Check sheet for the drawn part. Datum: minimum x, y, z corner. Units: mm. Coordinates: 2 decimals unless noted, no trailing zeros. Order: outer loops, then holes, each group sorted by start corner. A loop starts at its lowest first (then second) coordinate and runs counter-clockwise, first axis right, second up. Notation, with made-up numbers: (16.5, 11) - (69.5, 11) arc R30 ccw to (69.5, 36) - close; hole circle Ø2 at (82.25, -23). An arc over 180 degrees is marked (long way). Put each result on its own line as item: value.
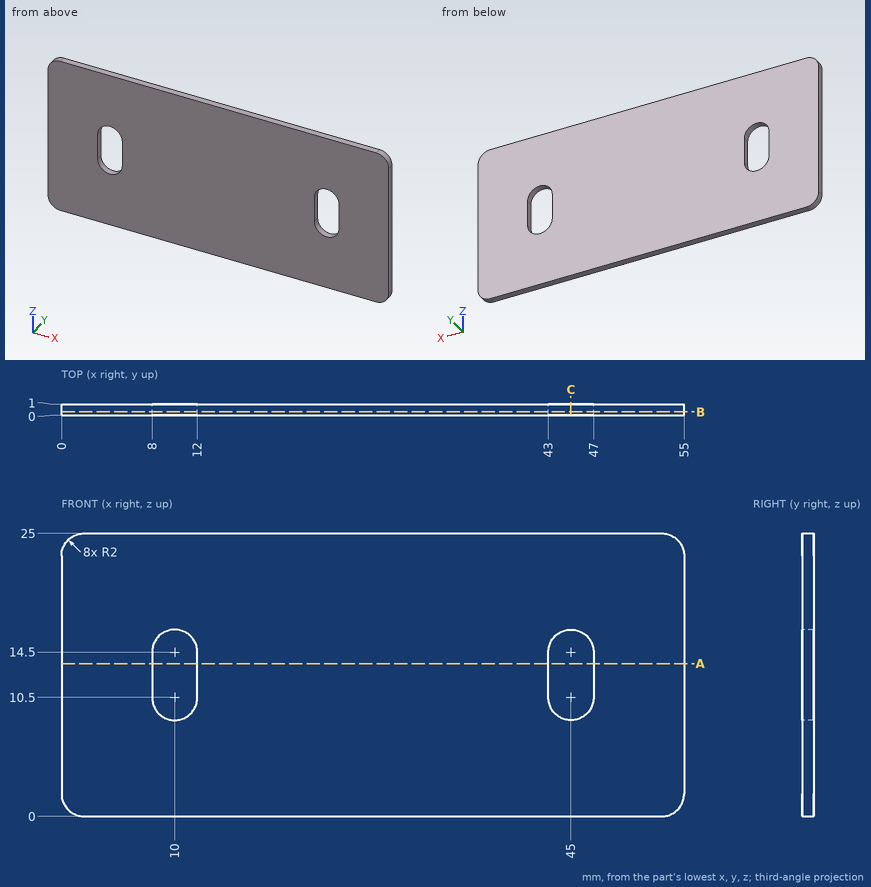
Q1. Section check A-A on z = 13.5. Record the boundary of the cut face in (x, y), then the cut area to 3 significant figures.
Answer block:
outline: (0, 0) - (8, 0) - (8, 1) - (0, 1) - close; (12, 0) - (43, 0) - (43, 1) - (12, 1) - close; (47, 0) - (55, 0) - (55, 1) - (47, 1) - close
area: 47.0 mm^2
Q2. Depth check by flat-ended pin: pin 1 Ø0.5 at (y, z) = (0.5, 13.5) entering from -X. Enter the tip coordinate at first touch or a pass-through.
Answer block:
pin 1: stops at x = 0
Q3. Section check B-B on y = 0.3. Record the boundary of the cut face in (x, z).
Answer block:
outline: (0, 2) arc R2 ccw to (2, 0) - (53, 0) arc R2 ccw to (55, 2) - (55, 23) arc R2 ccw to (53, 25) - (2, 25) arc R2 ccw to (0, 23) - close; hole (8, 10.5) arc R2 ccw to (12, 10.5) - (12, 14.5) arc R2 ccw to (8, 14.5) - close; hole (43, 10.5) arc R2 ccw to (47, 10.5) - (47, 14.5) arc R2 ccw to (43, 14.5) - close
Q4. Section check C-C on x = 45. Record the boundary of the cut face in (y, z), then the cut area to 3 significant figures.
Answer block:
outline: (0, 0) - (1, 0) - (1, 8.5) - (0, 8.5) - close; (0, 16.5) - (1, 16.5) - (1, 25) - (0, 25) - close
area: 17.0 mm^2
Q5. Thickness scan on L1, parallel to X at y = 0.15, z = 12.5; L2, parallel to X at y = 0.25, z = 16; L3, parallel to X at y = 0.2, z = 1.75. Record the ranges inside material, lowest first. Write a range as [from, to].
Answer block:
L1: x = [0, 8], [12, 43], [47, 55]
L2: x = [0, 8.68], [11.32, 43.68], [46.32, 55]
L3: x = [0.02, 54.98]
